Source: CAD feature listing. Evaluate the final solid. Frame: model axes, mm. Round coordinates to 2 decimals unless told otherwise and drop trailing zeros. Order: outer loops, then holes, each group sorted by start corner. A loop starts at its lowest first (then second) coordinate and runs counter-clockwise, first axis right, second up. Notation, with made-up numbers: (38, 84) -> (56, 84) arc R15 cw to (56, 113) -> close; hole circle Ø7 at (60.5, 32.5). An arc over 180 degrees is marked (long way). Write item = value, one per line. Start each with the question number.
(1) Ray query, line 1 (X direction, y = 50, z = -5.35); line 2 (X direction, y = -48.5, z = -6.7). Return the intervals inside material, ascending.
(2) Draft query along X for faces 1 (the face through (-1, 1, -7.2)), 2 (the face through (40.836, 48.663, -6.214)). Return one class per face: released by +X, released by -X, zero draft, split by the parting line, or undercut.
(3) Cut plane A-A on x = -37. Return the cut outline in (y, z).
(4) Cut plane B-B on x = 38. Return the cut outline in (y, z).
from build123d import *

# Parameters (mm, degrees)
SKETCH015_W     = 123.1
SKETCH015_H     = 111.7
PAD003_DEPTH    = 2
SKETCH020_R     = 4.4
POCKET010_DEPTH = 2.2
SKETCH021_R     = 4.4
POCKET011_DEPTH = 5.71
SKETCH022_R     = 4.4
POCKET012_DEPTH = 5.71


with BuildPart() as part:
    # Sketch015 → Pad003 (new body)
    with BuildSketch(Plane.XY.offset(-7.2)):
        Rectangle(SKETCH015_W, SKETCH015_H)
    extrude(amount=PAD003_DEPTH)

    # Sketch020 → Pocket010 (cut)
    with BuildSketch(Plane.XY.offset(-7.2)):
        with Locations((-36.708672, -51.151615)):
            Circle(SKETCH020_R)
    extrude(amount=POCKET010_DEPTH, mode=Mode.SUBTRACT)

    # Sketch021 → Pocket011 (cut)
    with BuildSketch(Plane(origin=(-2, 79.9, -7.2), x_dir=(1, 0, 0), z_dir=(0, 0, 1))):
        with Locations((-36.708672, -51.151615)):
            Circle(SKETCH021_R)
    extrude(amount=POCKET011_DEPTH, mode=Mode.SUBTRACT)

    # Sketch022 → Pocket012 (cut)
    with BuildSketch(Plane(origin=(73.48, 101.5, -7.2), x_dir=(1, 0, 0), z_dir=(0, 0, 1))):
        with Locations((-36.708672, -51.151615)):
            Circle(SKETCH022_R)
    extrude(amount=POCKET012_DEPTH, mode=Mode.SUBTRACT)


solid = part.part
Evaluation:
q1.line_1 = -61.55 to 32.39, 41.16 to 61.55
q1.line_2 = -61.55 to -40.22, -33.2 to 61.55
q2.face_1 = zero draft
q2.face_2 = undercut
q3.outline = (-55.85, -7.2) -> (-55.54, -7.2) -> (-55.54, -5.2) -> (-55.85, -5.2) -> close; (-46.76, -7.2) -> (24.69, -7.2) -> (24.69, -5.2) -> (-46.76, -5.2) -> close; (32.8, -7.2) -> (55.85, -7.2) -> (55.85, -5.2) -> (32.8, -5.2) -> close
q4.outline = (-55.85, -7.2) -> (46.12, -7.2) -> (46.12, -5.2) -> (-55.85, -5.2) -> close; (54.57, -7.2) -> (55.85, -7.2) -> (55.85, -5.2) -> (54.57, -5.2) -> close
